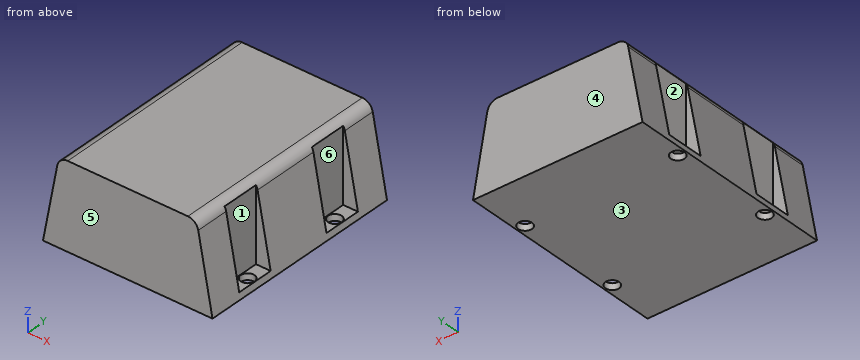
from build123d import *

# Parameters (mm, degrees)
SKETCH_1_W               = 80
SKETCH_1_H               = 100
EXTRUDE_1_DEPTH          = 40
SKETCH_2_OUTSIDE_W       = 108.832
SKETCH_2_OUTSIDE_H       = 68.832
CUT_EXTRUDE_1_DEPTH      = 1
CUT_EXTRUDE_1_DEPTH_BACK = 101
CUT_EXTRUDE_2_DEPTH      = 37
SKETCH_4_R               = 3.25
CUT_EXTRUDE_3_DEPTH      = 37
SKETCH_5_OUTSIDE_W       = 108.832
SKETCH_5_OUTSIDE_H       = 68.832
CUT_EXTRUDE_4_DEPTH      = 100


with BuildPart() as part:
    # 草图1 → 凸台-拉伸1 (new body)
    with BuildSketch(Plane.XY):
        Rectangle(SKETCH_1_W, SKETCH_1_H)
    extrude(amount=EXTRUDE_1_DEPTH)

    # 草图2 outside → 切除-拉伸1 (cut, two sides)
    with BuildSketch(Plane(origin=(0, -50, 0), x_dir=(-1, 0, 0), z_dir=(0, -1, 0))) as cut_extrude_1_sk:
        with Locations((0, -20)):
            Rectangle(SKETCH_2_OUTSIDE_W, SKETCH_2_OUTSIDE_H)
        Polygon((0, -40), (32.5, -40), (40, 0), (-40, 0), (-32.5, -40), align=None, mode=Mode.SUBTRACT)
    extrude(amount=CUT_EXTRUDE_1_DEPTH, mode=Mode.SUBTRACT)
    extrude(cut_extrude_1_sk.sketch, amount=-CUT_EXTRUDE_1_DEPTH_BACK, mode=Mode.SUBTRACT)

    # 草图3 → 切除-拉伸2 (cut)
    with BuildSketch(Plane.XY.offset(40)):
        Polygon((-40, -25), (-40, -34), (-32.5, -34), (-32.5, -16), (-40, -16), align=None)
        Polygon((-40, 16), (-40, 25), (-40, 34), (-32.5, 34), (-32.5, 16), align=None)
        Polygon((40, -16), (40, -25), (40, -34), (32.5, -34), (32.5, -16), align=None)
        Polygon((40, 25), (40, 34), (32.5, 34), (32.5, 16), (40, 16), align=None)
    extrude(amount=-CUT_EXTRUDE_2_DEPTH, mode=Mode.SUBTRACT)

    # 草图4 → 切除-拉伸3 (cut)
    with BuildSketch(Plane.XY.offset(3)):
        with Locations((-36, 25)):
            Circle(SKETCH_4_R)
        with Locations((36, 25)):
            Circle(SKETCH_4_R)
        with Locations((36, -25)):
            Circle(SKETCH_4_R)
        with Locations((-36, -25)):
            Circle(SKETCH_4_R)
    extrude(amount=-CUT_EXTRUDE_3_DEPTH, mode=Mode.SUBTRACT)

    # 草图5 outside → 切除-拉伸4 (cut)
    with BuildSketch(Plane.XZ.offset(50)):
        with Locations((0, 20)):
            Rectangle(SKETCH_5_OUTSIDE_W, SKETCH_5_OUTSIDE_H)
        with BuildLine():
            Line((-28.350368564, 40), (28.350368564, 40))
            ThreePointArc((28.350368564, 40), (31.543547749, 38.847545541), (33.264729498, 35.921442675))
            Line((33.264729498, 35.921442675), (40, 0))
            Line((40, 0), (-40, 0))
            Line((-40, 0), (-33.264729498, 35.921442675))
            ThreePointArc((-33.264729498, 35.921442675), (-31.543547749, 38.847545541), (-28.350368564, 40))
        make_face(mode=Mode.SUBTRACT)
    extrude(amount=-CUT_EXTRUDE_4_DEPTH, mode=Mode.SUBTRACT)


solid = part.part
Geometry check sheet. Reference: the model listing, model coordinates, mm. Face numbers are marked on the shaded views. A direction names the side the tool comes from. Give positions to 0.01 mm unless a question says otherwise; leave off trailing zeros. Loops run counter-clockwise (first coordinate to the right, second up) from the corner with the lowest first, then second, coordinate; pieces in that order, holes last. Notation, with made-up numbers: M 35.5,51.25 L 63.5,51.25 A32 ccw 63.5,87.25 Z; hole C -35,52.5 d4. An arc over 180 degrees is marked long. Answer as a JSON object with one key per item and string values. Group by question number.
Item 1: Sectioned sample at D-D on y = -40.5. Record the boundary of the cut face in (x, z).
Item 2: Sectioned sample at B-B on x = 36. Record the boundary of the cut face in (y, z), plus the area to 3 significant figures.
Item 3: Gauge pin test, flat ends, axial feed: pin 1 (6 mm diameter, centred on y = -19.5, z = 32, fed in from +X); pin 2 (4 mm diameter, centred on x = 36, y = -25, fed in from -Z); pin 3 (8 mm diameter, centred on y = 18.5, z = 19.5, fed in from -X); pin 4 (10.5 mm diameter, centred on x = 36, y = 25, fed in from +Z). Record the tip position at first contact, or that the pin passes through.
Item 4: Material ranges on L1, parallel to Y at x = 36, z = 1.7; L2, parallel to X at y = 20.5, z = 21.5; L3, parallel to X at y = 1.5, z = 2.5, recorded low to high.
Item 5: Sectioned sample at C-C on z = 6. Record the boundary of the cut face in (x, y) (3 decimals), plus the area to 3 significant figures.
Item 6: Sectioned sample at A-A on y = -25. Record the boundary of the cut face in (x, z).
Item 7: Access from +Z, -Z, +X, -X, +Y, -Y to the whole of each face (thin tool, end or side, straight path). Record for the marked faces 1, 2 and 3.
Item 8: Mould release check, pull along Y, two halves, no side actions. Record for the marked faces 4, 5 and 6: pulls with the +Y half, pulls with the -Y half, needs draft (parallel to the pull), parting line crosses it, or undercut.
Findings below:
{
 "1": {"outline": "M -40,0 L 40,0 L 33.26,35.92 A5 ccw 28.35,40 L -28.35,40 A5 ccw -33.26,35.92 Z"},
 "2": {"outline": "M -50,0 L -28.25,0 L -28.25,3 L -34,3 L -34,21.33 L -50,21.33 Z; M -21.75,0 L 21.75,0 L 21.75,3 L 16,3 L 16,21.33 L -16,21.33 L -16,3 L -21.75,3 Z; M 28.25,0 L 50,0 L 50,21.33 L 34,21.33 L 34,3 L 28.25,3 Z", "area": "1,430 mm2"},
 "3": {"pin 1": "x = 32.5", "pin 2": "through", "pin 3": "x = -36.93", "pin 4": "z = 39.39"},
 "4": {"L1": "-50 to -28.25, -21.75 to 21.75, 28.25 to 50", "L2": "-32.5 to 32.5", "L3": "-39.53 to 39.53"},
 "5": {"outline": "M -38.875,-50 L 38.875,-50 L 38.875,-34 L 32.5,-34 L 32.5,-16 L 38.875,-16 L 38.875,16 L 32.5,16 L 32.5,34 L 38.875,34 L 38.875,50 L -38.875,50 L -38.875,34 L -32.5,34 L -32.5,16 L -38.875,16 L -38.875,-16 L -32.5,-16 L -32.5,-34 L -38.875,-34 Z", "area": "7,320 mm2"},
 "6": {"outline": "M -40,0 L -39.25,0 L -39.25,3 L -39.44,3 Z; M -32.75,0 L 32.75,0 L 32.75,3 L 32.5,3 L 32.5,37.79 A5 ccw 28.35,40 L -28.35,40 A5 ccw -32.5,37.79 L -32.5,3 L -32.75,3 Z; M 39.25,0 L 40,0 L 39.44,3 L 39.25,3 Z"},
 "7": {"face 1": "+Z, +X", "face 2": "+Z, -X", "face 3": "-Z, +X, -X, +Y, -Y"},
 "8": {"face 4": "pulls with the +Y half", "face 5": "pulls with the -Y half", "face 6": "undercut"}
}
